Verification items for the finished model (mm, model axes). Round coordinates to 2 decimals unless told otherwise and drop trailing zeros. Write each loop counter-clockwise with the first axis right and the second up, starting at its lowest first coordinate (ties: lowest second). Pieces come first, ordered by that corner, then holes. Notation, with made-up numbers: M 61,5 L 101,5 A23 ccw 101,44 Z; hole C 59.5,-8 d7. An arc over 180 degrees is marked long. One line per question, with ' | ' between items. Start each with the question number.
Q1. Gauge pin test, flat ends, axial feed: pin 1 (1 mm diameter, centred on y = 7, z = 0.5, fed in from +X); pin 2 (1 mm diameter, centred on x = -4, z = 0.5, fed in from -Y). Record the tip position at first contact, or that the pin passes through.
Q2. Cross-section at A-A (x = 0). Record the boundary of the cut face in (y, z).
Q3. Release check for a two-part mould opening along X. For faces 1 (the face through (-9.676, -4.571, 1.479)), 2 (the face through (11.61, 11.45, 1.48)), 3 (the face through (-12.21, 11.95, 1.48)), 4 (the face through (0, 5, 0)) record: released by +X, released by -X, zero draft, split by the parting line, or undercut.
Q4. Cross-section at D-D (z = 2.5). Record the boundary of the cut face in (x, y), then the cut area to 3 significant figures.
Q5. Thickness scan on line 1 along X through (y, z) = (14, 0.5); line 2 along Y through (x, z) = (0, 2); line 3 along Y through (x, z) = (0.5, 2.5). Record the ranges inside material, lowest first. Write a range as from..to.
Q6. Cross-section at C-C (x = -10). Record the boundary of the cut face in (y, z), then the cut area to 3 significant figures.
Q7. Cross-section at B-B (y = -14.5). Record the boundary of the cut face in (x, z).
Autodesk Inventor part; units mm, degrees
ref_plane "Work Plane4" through (-10, 13.9812, 0) normal (1, 0, 0) x (0, 0, -1)
ref_plane "Work Plane12" through (-10, 14.4812, 0) normal (0, 1, 0) x (1, 0, 0)
ref_plane "YZ Plane" through (0, 0, 0) normal (1, 0, 0) x (0, 1, 0)
sketch "Sketch1" plane through (0, 0, 0) normal (0, 0, 1) x (1, 0, 0)
  circle A0 centre (-10, 13.9812) radius 3
  circle A1 centre (10, 13.9812) radius 3
  circle A2 centre (0, -4.0188) radius 2.5
  circle A3 centre (0, -14.0188) radius 2.5
  line L0 (-1.6291, -18.508) -> (1.6291, -18.508)
  line L1 (-17.5, 8.9812) -> (-1.6291, -18.508)
  line L2 (-17.5, 8.9812) -> (17.1989, 8.9812) construction
  line L3 (17.5, 8.9812) -> (1.6291, -18.508)
  line L4 (17.5, 8.9812) -> (62.1106, 8.9812) construction
  line L5 (-17.5, 8.9812) -> (-17.5, 18.9812)
  line L6 (-17.5, 18.9812) -> (17.5, 18.9812)
  line L7 (17.5, 18.9812) -> (17.5, 8.9812)
  point P0 (0, -18.508)
  dimension "d1" = 5
  dimension "d2" = 10
  dimension "d3" = 6
  dimension "d4" = 10
  dimension "d5" = 60
  dimension "d10" = 35
  dimension "d11" = 17.5
  dimension "d13" = 3.2582
  dimension "d17" = 120
  dimension "d20" = 10
  dimension "d22" = 23
  dimension "d26" = 5
extrude "Extrusion1" add sketch "Sketch1" along normal blind 3
ref_plane "Work Plane4" through (-10, 13.9812, 0) normal (1, 0, 0) x (0, 0, -1)
ref_plane "Work Plane1" through (-13, 13.9812, 0) normal (-1, 0, 0) x (0, 0, 1)
ref_plane "Work Plane3" through (-7, 13.9812, 0) normal (1, 0, 0) x (0, 0, -1)
mirror "Mirror1" about plane through (0, 0, 0) normal (1, 0, 0)
ref_plane "Work Plane10" through (-10, 16.9812, 0) normal (0, 1, 0) x (1, 0, 0)
ref_plane "Work Plane12" through (-10, 14.4812, 0) normal (0, 1, 0) x (1, 0, 0)
ref_plane "Work Plane11" through (-10, 11.9812, 0) normal (0, 1, 0) x (1, 0, 0)
ref_plane "Work Plane5" through (10, 13.9812, 0) normal (1, 0, 0) x (0, 0, -1)
equation "\"d11\" = 0.5 * d10"
properties part number "Load Cell Connector to Extrusion Bar"
Determined:
1) pin 1: stops at x = 16.64 | pin 2: stops at y = -15.27
2) outline: M -18.51,0 L -16.52,0 L -16.52,3 L -18.51,3 Z; M -11.52,0 L -6.52,0 L -6.52,3 L -11.52,3 Z; M -1.52,0 L 18.98,0 L 18.98,3 L -1.52,3 Z
3) face 1: released by -X | face 2: undercut | face 3: undercut | face 4: zero draft
4) outline: M -17.5,8.98 L -1.63,-18.51 L 1.63,-18.51 L 17.5,8.98 L 17.5,18.98 L -17.5,18.98 Z; hole C -10,13.98 d6; hole C 0,-14.02 d5; hole C 0,-4.02 d5; hole C 10,13.98 d6 | area: 780 mm²
5) line 1: x = -17.5..-13, -7..7, 13..17.5 | line 2: y = -18.51..-16.52, -11.52..-6.52, -1.52..18.98 | line 3: y = -18.51..-16.47, -11.57..-6.47, -1.57..18.98
6) outline: M -4.01,0 L 10.98,0 L 10.98,3 L -4.01,3 Z; M 16.98,0 L 18.98,0 L 18.98,3 L 16.98,3 Z | area: 51.0 mm²
7) outline: M -3.94,0 L -2.45,0 L -2.45,3 L -3.94,3 Z; M 2.45,0 L 3.94,0 L 3.94,3 L 2.45,3 Z
